Build history of the part. All positions in model axes, mm. Give positions to 0.01 mm unless a question says otherwise; leave off trailing zeros. Order: outer loops, then holes, each group sorted by start corner. A loop starts at its lowest first (then second) coordinate and runs counter-clockwise, first axis right, second up. Notation, with made-up numbers: (51, 3.5) - (67, 3.5) arc R31 ccw to (67, 30.5) - close; hole circle Ø5 at (5, 63). An arc over 180 degrees is marked (long way). Answer in a Markdown table with one row per item.
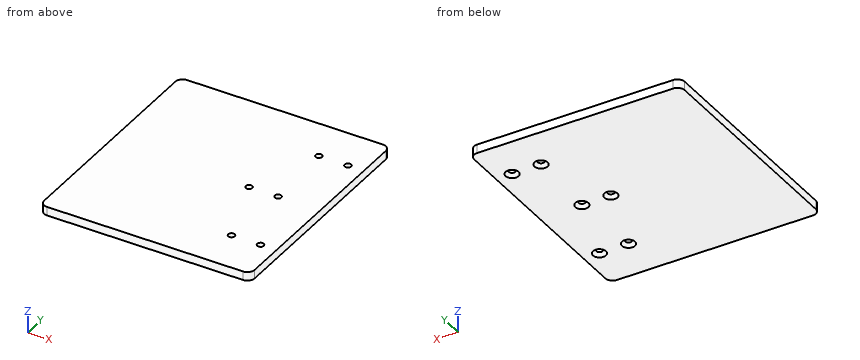
Solid Edge part; units mm, degrees
sketch "Sketch1" plane through (60.3162, 60.3162, 0) normal (0, 0, 1) x (1, 0, 0)
  line L0 (-132.8162, -140.3162) -> (12.1838, -140.3162)
  line L1 (12.1838, -140.3162) -> (12.1838, 19.6838)
  line L2 (12.1838, 19.6838) -> (-132.8162, 19.6838)
  line L3 (-132.8162, 19.6838) -> (-132.8162, -140.3162)
  dimension "D1" = 12.1838
  dimension "D2" = 12.1838
extrude "Protrusion1" add sketch "Sketch1" against normal blind 6
fillet "Verrundung_1" radius 5 4 edges at (-72.5, 80, -3) (72.5, 80, -3) (72.5, -80, -3) (-72.5, -80, -3)
hole "Bohrung_3" at (43.5, 0, -6) direction (0, 0, 1) diameter 4.5 end up to next countersink diameter 9 countersink angle 90
hole "Hole1" at (23.5, 0, -6) direction (0, 0, 1) diameter 4.5 end up to next countersink diameter 9 countersink angle 90
hole "Bohrung_5" at (61.5, -50, -6) direction (0, 0, 1) diameter 4.5 end up to next countersink diameter 9 countersink angle 90
hole "Hole2" at (41.5, -50, -6) direction (0, 0, 1) diameter 4.5 end up to next countersink diameter 9 countersink angle 90
mirror "Mirror1" about plane through (9.6062, 0, 9.6062) normal (0, -1, 0) of "Bohrung_5", "Hole2"
properties material "Aluminium, 1060"
1. Drop flat-ended pins along their axis: P1, Ø5, axis at x = 41.5, y = 50, coming from the -Z side; P2, Ø1, axis at x = 41.5, y = 49.5, coming from the +Z side. Give the stop position or say it passes through.
Check result:
| item | result |
|---|---|
| P1 | stops at z = -4 |
| P2 | passes through |
2. Cut at C-C on x = 61.5. Write the cut outline in (y, z).
Check result:
| item | result |
|---|---|
| outline | (-80, -6) - (-54.5, -6) - (-52.25, -3.75) - (-52.25, 0) - (-80, 0) - close; (-47.75, -3.75) - (-45.5, -6) - (45.5, -6) - (47.75, -3.75) - (47.75, 0) - (-47.75, 0) - close; (52.25, -3.75) - (54.5, -6) - (80, -6) - (80, 0) - (52.25, 0) - close |
3. Probe line 1 (X direction, y = 50, z = -0.85); line 2 (X direction, y = 0, z = -1.7); line 3 (Y direction, x = 61.5, z = -1.4). List the from-to ranges inside material, lowest first.
Check result:
| item | result |
|---|---|
| line 1 | x = -72.5 to 39.25, 43.75 to 59.25, 63.75 to 72.5 |
| line 2 | x = -72.5 to 21.25, 25.75 to 41.25, 45.75 to 72.5 |
| line 3 | y = -80 to -52.25, -47.75 to 47.75, 52.25 to 80 |
4. Cut at A-A on y = 0. Write the cut outline in (x, z).
Check result:
| item | result |
|---|---|
| outline | (-72.5, -6) - (19, -6) - (21.25, -3.75) - (21.25, 0) - (-72.5, 0) - close; (25.75, -3.75) - (28, -6) - (39, -6) - (41.25, -3.75) - (41.25, 0) - (25.75, 0) - close; (45.75, -3.75) - (48, -6) - (72.5, -6) - (72.5, 0) - (45.75, 0) - close |
5. Cut at B-B on x = 23.5. Write the cut outline in (y, z), and give its area (3 significant figures).
Check result:
| item | result |
|---|---|
| outline | (-80, -6) - (-4.5, -6) - (-2.25, -3.75) - (-2.25, 0) - (-80, 0) - close; (2.25, -3.75) - (4.5, -6) - (80, -6) - (80, 0) - (2.25, 0) - close |
| area | 928 mm² |
